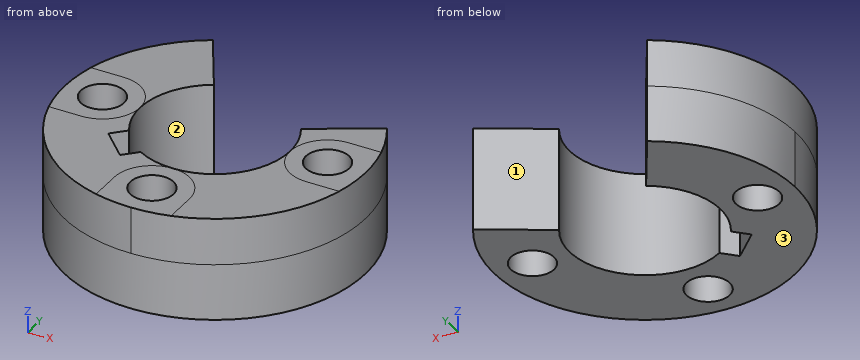
from build123d import *
from build123d.topology import SkipClean

# Parameters (mm, degrees)
SKETCH1_R           = 1.15
BOSS_EXTRUDE1_DEPTH = 8
SKETCH4_R           = 8
SKETCH4_R_2         = 1.15
BOSS_EXTRUDE2_DEPTH = 3
CUT_EXTRUDE3_DEPTH  = 5.5
SKETCH6_R           = 42
CUT_EXTRUDE5_DEPTH  = 5.5
SKETCH5_R           = 1.15
CUT_EXTRUDE6_DEPTH  = 50.185871955


with BuildPart() as part:
    # Sketch1 → Boss-Extrude1 (new body)
    with BuildSketch(Plane.XY):
        with BuildLine():
            Line((0, -42), (0, -40))
            ThreePointArc((0, -40), (22.793187837, -20.077432085), (6.099520657, 5.176470588))
            ThreePointArc((6.099520657, 5.176470588), (7.259881704, -3.360672202), (0, -8))
            ThreePointArc((0, -8), (-8, 0), (0, 8))
            ThreePointArc((0, 8), (25, -17), (0, -42))
        make_face()
        with Locations((0, 6)):
            Circle(SKETCH1_R, mode=Mode.SUBTRACT)
        with Locations((-6, 0)):
            Circle(SKETCH1_R, mode=Mode.SUBTRACT)
        with Locations((0, -6)):
            Circle(SKETCH1_R, mode=Mode.SUBTRACT)
        with Locations((6, 0)):
            Circle(SKETCH1_R, mode=Mode.SUBTRACT)
    extrude(amount=BOSS_EXTRUDE1_DEPTH)

    # Sketch4 → Boss-Extrude2 (add)
    with SkipClean():  # the faces are left unmerged after this step: merging them gives an invalid solid
        with BuildSketch(Plane(origin=(0, 0, 0), x_dir=(-1, 0, 0), z_dir=(0, 0, -1))):
            Circle(SKETCH4_R)
            with Locations((0, 6)):
                Circle(SKETCH4_R_2, mode=Mode.SUBTRACT)
            with Locations((-6, 0)):
                Circle(SKETCH4_R_2, mode=Mode.SUBTRACT)
            with Locations((0, -6)):
                Circle(SKETCH4_R_2, mode=Mode.SUBTRACT)
            with Locations((6, 0)):
                Circle(SKETCH4_R_2, mode=Mode.SUBTRACT)
        extrude(amount=BOSS_EXTRUDE2_DEPTH)

    # Sketch3 → Cut-Extrude3 (cut)
    with SkipClean():  # the faces are left unmerged after this step: merging them gives an invalid solid
        with BuildSketch(Plane.XY.offset(8)):
            with BuildLine():
                Line((6, 2), (10, 2))
                Line((10, 2), (10, -2))
                Line((10, -2), (6, -2))
                ThreePointArc((6, -2), (4, 0), (6, 2))
            make_face()
            with BuildLine():
                Line((2, -6), (2, -10))
                Line((2, -10), (-2, -10))
                Line((-2, -10), (-2, -6))
                ThreePointArc((-2, -6), (0, -4), (2, -6))
            make_face()
            with BuildLine():
                Line((-6, -2), (-10, -2))
                Line((-10, -2), (-10, 2))
                Line((-10, 2), (-6, 2))
                ThreePointArc((-6, 2), (-4, 0), (-6, -2))
            make_face()
            with BuildLine():
                Line((-2, 6), (-2, 10))
                Line((-2, 10), (2, 10))
                Line((2, 10), (2, 6))
                ThreePointArc((2, 6), (0, 4), (-2, 6))
            make_face()
        extrude(amount=-CUT_EXTRUDE3_DEPTH, mode=Mode.SUBTRACT)

    # Sketch6 → Cut-Extrude5 (cut)
    with SkipClean():  # the faces are left unmerged after this step: merging them gives an invalid solid
        with BuildSketch(Plane.XY.offset(8)):
            Circle(SKETCH6_R)
        extrude(amount=-CUT_EXTRUDE5_DEPTH, mode=Mode.SUBTRACT)

    # Sketch5 → Cut-Extrude6 (cut, through all)
    with BuildSketch(Plane(origin=(0, 0, -3), x_dir=(-1, 0, 0), z_dir=(0, 0, -1))):
        with BuildLine():
            Line((-6.92820323, 4), (-3.464101615, 2))
            ThreePointArc((-3.464101615, 2), (-2.815501367, -2.84129408), (2.031506006, -3.445719569))
            Line((2.031506006, -3.445719569), (2.738612788, -4.15282635))
            Line((2.738612788, -4.15282635), (4.15282635, -2.738612788))
            Line((4.15282635, -2.738612788), (3.445719569, -2.031506006))
            ThreePointArc((3.445719569, -2.031506006), (3.868383537, 1.017648668), (2, 3.464101615))
            Line((2, 3.464101615), (4, 6.92820323))
            ThreePointArc((4, 6.92820323), (-2.070552361, 7.72740661), (-6.92820323, 4))
        make_face()
        with Locations((0, 6)):
            Circle(SKETCH5_R, mode=Mode.SUBTRACT)
    extrude(amount=-CUT_EXTRUDE6_DEPTH, mode=Mode.SUBTRACT)


with BuildPart() as cut_extrude6_kept_piece:
    # of the separate pieces the step leaves, the one the design keeps (cut_extrude6_pieces_kept)
    add(part.part.solids().sort_by_distance((-4, 6.92820323, -3))[0])


solid = cut_extrude6_kept_piece.part
The model under review builds one solid part; all positions refer to its coordinate system, in mm. Face numbers are marked on the shaded views. Round coordinates to 2 decimals unless told otherwise and drop trailing zeros. Loops run counter-clockwise (first coordinate to the right, second up) from the corner with the lowest first, then second, coordinate; pieces in that order, holes last. Notation, with made-up numbers: (-4, 6.25) - (6, 6.25) arc R34 ccw to (6, 37.25) - close; hole circle Ø3 at (2, 89.25). An arc over 180 degrees is marked (long way). Use CSV: the item, a comma, the result in double quotes.
(1) The part is to be moulded in two halves that separate along Y. For the marked faces 1, 2 and 3, say which applies: pulls with the +Y half, pulls with the -Y half, needs draft (parallel to the pull), parting line crosses it, or undercut.
Working result:
face 1,"pulls with the +Y half"
face 2,"undercut"
face 3,"needs draft"
(2) Take a section at A-A, the plane y = -3.75. Give the boundary of the cut face in (x, z), plus the area to 3 significant figures.
Working result:
outline,"(-7.07, -3) - (-3.14, -3) - (-3.14, 2.5) - (-7.07, 2.5) - close; (-2.34, -3) - (-1.39, -3) - (-1.39, 2.5) - (-2.34, 2.5) - close; (1.39, -3) - (7.07, -3) - (7.07, 2.5) - (1.39, 2.5) - close"
area,"58.0 mm^2"
(3) Take a section at C-C, the plane x = -5.25. Give the boundary of the cut face in (y, z), plus the area to 3 significant figures.
Working result:
outline,"(-6.04, -3) - (-0.87, -3) - (-0.87, 2.5) - (-6.04, 2.5) - close; (0.87, -3) - (6.04, -3) - (6.04, 2.5) - (0.87, 2.5) - close"
area,"56.8 mm^2"
(4) Take a section at B-B, the plane z = 0.7. Give the boundary of the cut face in (x, y).
Working result:
outline,"(-4.15, -2.74) - (-3.45, -2.03) arc R4 cw to (-2, 3.46) - (-4, 6.93) arc R8 ccw (long way) to (6.93, 4) - (3.46, 2) arc R4 cw to (-2.03, -3.45) - (-2.74, -4.15) - close; hole circle Ø2.3 at (-6, 0); hole circle Ø2.3 at (0, -6); hole circle Ø2.3 at (6, 0)"
(5) Clearance check with flat-ended pins moving along their axes: P1, Ø3, axis at y = 4, z = 1, coming from the -X side; P2, Ø1.4, axis at x = -6, y = 0, coming from the +Z side; P3, Ø2, axis at x = 5, z = 0.5, coming from the +Y side. State where each tip first meets the part, or that it passes through.
Working result:
P1,"stops at x = -7.6"
P2,"passes through"
P3,"stops at y = 3.46"
(6) Take a section at D-D, the plane y = -6. Give the boundary of the cut face in (x, z), plus the area to 3 significant figures.
Working result:
outline,"(-5.29, -3) - (-1.15, -3) - (-1.15, 2.5) - (-5.29, 2.5) - close; (1.15, -3) - (5.29, -3) - (5.29, 2.5) - (1.15, 2.5) - close"
area,"45.6 mm^2"
(7) For line 1 (X direction, y = 0, z = 1.4); line 2 (X direction, y = 1, z = 0.05); line 3 (X direction, y = -5, z = -2.25) (3 decimals), list the stretches that pass through material, from the lowest coordinate up.
Working result:
line 1,"x = -8 to -7.15, -4.85 to -4, 4 to 4.85, 7.15 to 8"
line 2,"x = -7.94 to -6.57, -5.43 to -3.87, 3.87 to 5.43, 6.57 to 7.94"
line 3,"x = -6.245 to -0.568, 0.568 to 6.245"
